Verification items for the finished model (mm, model axes). A direction names the side the tool comes from. Give positions to 0.01 mm unless a question says otherwise; leave off trailing zeros. Order: outer loops, then holes, each group sorted by start corner. A loop starts at its lowest first (then second) coordinate and runs counter-clockwise, first axis right, second up. Notation, with made-up numbers: (68, 71.5) -> (77, 71.5) arc R21 cw to (77, 95.5) -> close; hole circle Ø1 at (-18.5, 19). An arc over 180 degrees is marked (long way). Return JSON: item names as keys, results as strings. Group by question number.
(1) Cross-section at A-A on y = 0. Enter the section's corners in (x, z), then the cut area to 3 significant figures.
(2) Cross-section at B-B on x = 1. Enter the section's corners in (y, z), then the cut area to 3 significant figures.
(3) Tool access check on faces 1 (the face through (2.96, -5.22, 23.91)), 2 (the face through (-3, 5.4, 20.8)), 3 (the face through (-6, 0, 24)), 4 (the face through (-2.96, 5.22, 23.91)), 5 (the face through (3.042, 5.172, 23.906)). Record the directions out of +Z, -Z, +X, -X, +Y, -Y that give a thin tool (end or side, any length) a straight path to the whole face; none if there is none.
(4) Depth check by flat-ended pin: pin 1 Ø3 at (y, z) = (-4, 6.5) entering from +X; pin 2 Ø3 at (y, z) = (-5.5, 24) entering from -X; pin 3 Ø5 at (y, z) = (0, 23.5) entering from -X; pin 4 Ø2.5 at (x, y) = (0, 0) entering from +Z. Enter the tip coordinate at first touch or a pass-through.
(5) Cross-section at C-C on z = 2. Enter the section's corners in (x, y), then the cut area to 3 significant figures.
(6) Thickness scan on line 1 along X through (y, z) = (0, 12); line 2 along X through (y, z) = (1.75, 13). Record the ranges inside material, lowest first.
(7) Cross-section at D-D on y = -4.5. Enter the section's corners in (x, z).
(8) Release check for a two-part mould opening along X. For faces 6 (the face through (7.39, -3.06, 10.25)), 7 (the face through (6, 0, 24)), 8 (the face through (2.957, 0.931, 9.17)), 9 (the face through (-4.9, -1.5, 8)) record: pulls with the +X half, pulls with the -X half, needs draft (parallel to the pull), parting line crosses it, or undercut.
from build123d import *

# Parameters (mm, degrees)
CROQUIS1_R              = 8
CROQUIS1_R_2            = 3.1
SALIENTE_EXTRUIR1_DEPTH = 20.8
CROQUIS2_R              = 3.1
CROQUIS2_R_2            = 2
SALIENTE_EXTRUIR2_DEPTH = 2.2
CROQUIS3_R              = 2
SALIENTE_EXTRUIR3_DEPTH = 6.3
CORTAR_EXTRUIR1_REACH   = 10
CROQUIS4_R              = 2.5


with BuildPart() as part:
    # Croquis1 → Saliente-Extruir1 (new body)
    with BuildSketch(Plane.XY):
        Circle(CROQUIS1_R)
        Circle(CROQUIS1_R_2, mode=Mode.SUBTRACT)
    extrude(amount=SALIENTE_EXTRUIR1_DEPTH)

    # Croquis2 → Saliente-Extruir2 (add)
    with BuildSketch(Plane.XY.offset(20.8)):
        Circle(CROQUIS2_R)
        Circle(CROQUIS2_R_2, mode=Mode.SUBTRACT)
    extrude(amount=-SALIENTE_EXTRUIR2_DEPTH)

    # Croquis3 → Saliente-Extruir3 (add)
    with BuildSketch(Plane.XY.offset(20.8)):
        Polygon((0, 6.92820323), (-6, 3.464101615), (-6, -3.464101615), (0, -6.92820323), (6, -3.464101615), (6, 3.464101615), align=None)
        Circle(CROQUIS3_R, mode=Mode.SUBTRACT)
    extrude(amount=SALIENTE_EXTRUIR3_DEPTH)

    # Croquis4 → Cortar-Extruir1 (cut, up to next)
    with BuildSketch(Plane(origin=(0, 0, 0), x_dir=(0, 0, -1), z_dir=(1, 0, 0)), mode=Mode.PRIVATE) as cortar_extruir1_sk1:
        with Locations((-6, 0)):
            Circle(CROQUIS4_R)
    cortar_extruir1_tool1 = extrude(cortar_extruir1_sk1.sketch, amount=-CORTAR_EXTRUIR1_REACH, mode=Mode.PRIVATE) & part.part
    add(cortar_extruir1_tool1.solids().sort_by_distance((0, 0, 6))[0], mode=Mode.SUBTRACT)


solid = part.part
Verdict:
{
 "1": {"outline": "(-8, 0) -> (-3.1, 0) -> (-3.1, 3.5) -> (-8, 3.5) -> close; (-8, 8.5) -> (-3.1, 8.5) -> (-3.1, 18.6) -> (-2, 18.6) -> (-2, 27.1) -> (-6, 27.1) -> (-6, 20.8) -> (-8, 20.8) -> close; (2, 18.6) -> (3.1, 18.6) -> (3.1, 0) -> (8, 0) -> (8, 20.8) -> (6, 20.8) -> (6, 27.1) -> (2, 27.1) -> close", "area": "235 mm²"},
 "2": {"outline": "(-7.94, 0) -> (-2.93, 0) -> (-2.93, 18.6) -> (-1.73, 18.6) -> (-1.73, 27.1) -> (-6.35, 27.1) -> (-6.35, 20.8) -> (-7.94, 20.8) -> close; (1.73, 18.6) -> (2.93, 18.6) -> (2.93, 0) -> (7.94, 0) -> (7.94, 20.8) -> (6.35, 20.8) -> (6.35, 27.1) -> (1.73, 27.1) -> close", "area": "272 mm²"},
 "3": {"face 1": "+Z, +X, -Y", "face 2": "+Z", "face 3": "+Z, -X, +Y, -Y", "face 4": "+Z, -X, +Y", "face 5": "+Z, +X, +Y"},
 "4": {"pin 1": "x = 7.6", "pin 2": "x = -5.07", "pin 3": "x = -6", "pin 4": "through"},
 "5": {"outline": "circle Ø16 at (0, 0); hole circle Ø6.2 at (0, 0)", "area": "171 mm²"},
 "6": {"line 1": "-8 to -3.1, 3.1 to 8", "line 2": "-7.81 to -2.56, 2.56 to 7.81"},
 "7": {"outline": "(-6.61, 0) -> (6.61, 0) -> (6.61, 20.8) -> (4.21, 20.8) -> (4.21, 27.1) -> (-4.21, 27.1) -> (-4.21, 20.8) -> (-6.61, 20.8) -> close"},
 "8": {"face 6": "parting line crosses it", "face 7": "pulls with the +X half", "face 8": "undercut", "face 9": "needs draft"}
}
